Work out the finished part from the listing and answer in its coordinate system (mm). Round coordinates to 2 decimals unless told otherwise and drop trailing zeros. Loops run counter-clockwise (first coordinate to the right, second up) from the corner with the lowest first, then second, coordinate; pieces in that order, holes last.
```python
from build123d import *

# Parameters (mm, degrees)
SKETCH1_W           = 450
SKETCH1_H           = 103
BOSS_EXTRUDE1_DEPTH = 4
SKETCH6_R           = 7.5
CUT_EXTRUDE4_DEPTH  = 5
SKETCH7_R           = 7.5
CUT_EXTRUDE5_DEPTH  = 5
SKETCH8_R           = 1.75
CUT_EXTRUDE6_DEPTH  = 5
SKETCH10_W          = 3
SKETCH10_H          = 103
CUT_EXTRUDE7_DEPTH  = 10


with BuildPart() as part:
    # Sketch1 → Boss-Extrude1 (new body)
    with BuildSketch(Plane.XY):
        with Locations((225, 51.5)):
            Rectangle(SKETCH1_W, SKETCH1_H)
    extrude(amount=BOSS_EXTRUDE1_DEPTH)

    # Sketch6 → Cut-Extrude4 (cut, through all)
    with BuildSketch(Plane.XY.offset(4)):
        with Locations((50, 30)):
            Circle(SKETCH6_R)
    extrude(amount=-CUT_EXTRUDE4_DEPTH, mode=Mode.SUBTRACT)

    # Sketch7 → Cut-Extrude5 (cut, through all)
    with BuildSketch(Plane.XY.offset(4)):
        with Locations((420, 30)):
            Circle(SKETCH7_R)
    extrude(amount=-CUT_EXTRUDE5_DEPTH, mode=Mode.SUBTRACT)

    # Sketch8 → Cut-Extrude6 (cut, through all)
    with BuildSketch(Plane.XY.offset(4)):
        with Locations((435, 45)):
            Circle(SKETCH8_R)
        with Locations((405, 45)):
            Circle(SKETCH8_R)
        with Locations((405, 15)):
            Circle(SKETCH8_R)
        with Locations((435, 15)):
            Circle(SKETCH8_R)
    extrude(amount=-CUT_EXTRUDE6_DEPTH, mode=Mode.SUBTRACT)

    # Sketch10 → Cut-Extrude7 (cut)
    with BuildSketch(Plane(origin=(0, 0, 0), x_dir=(-1, 0, 0), z_dir=(0, 0, -1))):
        with Locations((-448.5, 51.5)):
            Rectangle(SKETCH10_W, SKETCH10_H)
    extrude(amount=-CUT_EXTRUDE7_DEPTH, mode=Mode.SUBTRACT)


solid = part.part
```
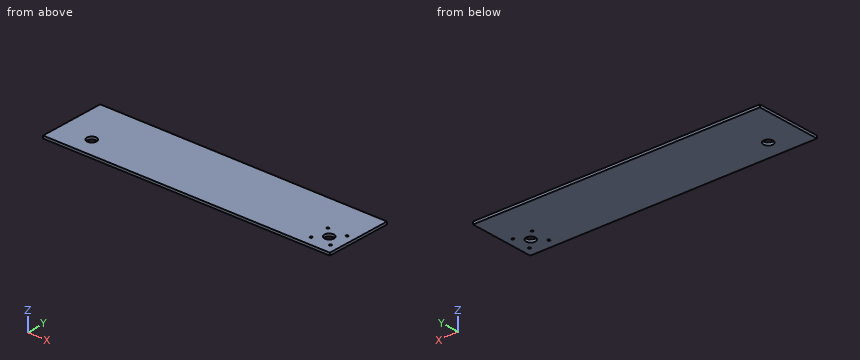
1. Consider probe 1 along Y at (x, z) = (435, 2.5); probe 2 along X at (y, z) = (31, 2.6); probe 3 along Y at (x, z) = (50, 1.9). Determine where each line is inside the solid, lowest interval first.
Answer key:
probe 1: y = 0 to 13.25, 16.75 to 43.25, 46.75 to 103
probe 2: x = 0 to 42.57, 57.43 to 412.57, 427.43 to 447
probe 3: y = 0 to 22.5, 37.5 to 103
2. Given pin 1 (1 mm diameter, centred on x = 105, y = 49.5, fed in from -Z); pin 2 (9 mm diameter, centred on x = 50, y = 30, fed in from -Z), each flat-ended and moving along its own axis, determine where each tip first touches the part or whether it passes through.
Answer key:
pin 1: stops at z = 0
pin 2: passes through
3. Find section B-B (x = 50). Write down the section's boundary in (y, z).
Answer key:
outline: (0, 0) - (22.5, 0) - (22.5, 4) - (0, 4) - close; (37.5, 0) - (103, 0) - (103, 4) - (37.5, 4) - close
4. Find section A-A (y = 30). Write down the section's boundary in (x, z).
Answer key:
outline: (0, 0) - (42.5, 0) - (42.5, 4) - (0, 4) - close; (57.5, 0) - (412.5, 0) - (412.5, 4) - (57.5, 4) - close; (427.5, 0) - (447, 0) - (447, 4) - (427.5, 4) - close
